from build123d import *

# Parameters (mm, degrees)
SKETCH2_W             = 50
SKETCH2_H             = 50
SKETCH2_R             = 9.525
BOSS_EXTRUDE1_DEPTH   = 6.35
F_4_CLEARANCE_HOLE1_D = 3.2639


with BuildPart() as part:
    # Sketch2 → Boss-Extrude1 (new body)
    with BuildSketch(Plane(origin=(0, 0, 0), x_dir=(1, 0, 0), z_dir=(0, 1, 0))):
        Rectangle(SKETCH2_W, SKETCH2_H)
        Circle(SKETCH2_R, mode=Mode.SUBTRACT)
    extrude(amount=BOSS_EXTRUDE1_DEPTH)

    # #4 Clearance Hole1 (through all)
    with Locations(Plane(origin=(0, 6.35, 0), x_dir=(1, 0, 0), z_dir=(0, 1, 0))):
        with Locations((-21, -21), (21, -21), (21, 21), (-21, 21)):
            Hole(F_4_CLEARANCE_HOLE1_D / 2)


solid = part.part
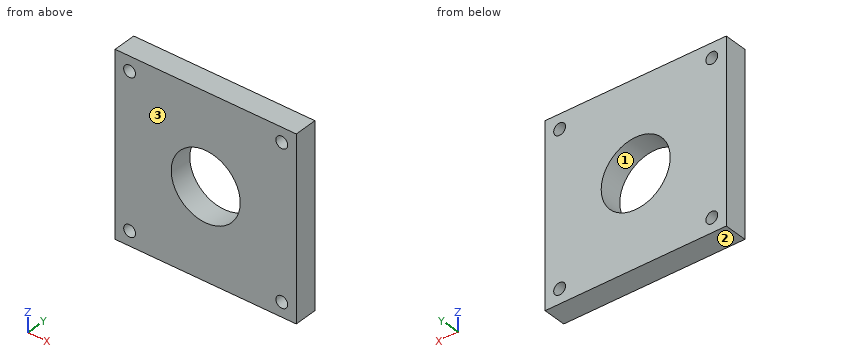
The listing builds one solid part. Answer for the finished solid, in the listing's coordinates (mm). Face numbers are marked on the shaded views. Round coordinates to 2 decimals unless told otherwise and drop trailing zeros. Order: outer loops, then holes, each group sorted by start corner. A loop starts at its lowest first (then second) coordinate and runs counter-clockwise, first axis right, second up. Notation, with made-up numbers: M 9.25,-33 L 65.25,-33 A21 cw 65.25,-6 Z; hole C 55.25,-11 d11. An arc over 180 degrees is marked long. Answer in a Markdown table with one row per item. Add a question column.
1) The part is cut by section C-C on x = 0. Determine the outline of the cut face in (y, z) (3 decimals), plus the area to 3 significant figures.
2) Consider line 1 along X through (y, z) = (2.5, 21); line 2 along Z through (x, y) = (0, 2.75) (3 decimals). Determine where each line is inside the solid, lowest interval first. Write a range as from..to.
3) The part is cut by section D-D on z = 0. Determine the outline of the cut face in (x, y) (3 decimals).
4) The part is cut by section A-A on z = 21. Determine the outline of the cut face in (x, y), plus the area to 3 significant figures.
5) Determine the mould class of the marked faces 1, 2 and 3 for opening direction Z: pulls with the +Z half, pulls with the -Z half, needs draft (parallel to the pull), parting line crosses it, or undercut.
6) The part is cut by section B-B on x = 21. Determine the outline of the cut face in (y, z), plus the area to 3 significant figures.
Findings below:
| question | item | result |
|---|---|---|
| 1 | outline | M 0,-25 L 6.35,-25 L 6.35,-9.525 L 0,-9.525 Z; M 0,9.525 L 6.35,9.525 L 6.35,25 L 0,25 Z |
| 1 | area | 197 mm² |
| 2 | line 1 | x = -25..-22.63, -19.37..19.37, 22.63..25 |
| 2 | line 2 | z = -25..-9.525, 9.525..25 |
| 3 | outline | M -25,0 L -9.525,0 L -9.525,6.35 L -25,6.35 Z; M 9.525,0 L 25,0 L 25,6.35 L 9.525,6.35 Z |
| 4 | outline | M -25,0 L -22.63,0 L -22.63,6.35 L -25,6.35 Z; M -19.37,0 L 19.37,0 L 19.37,6.35 L -19.37,6.35 Z; M 22.63,0 L 25,0 L 25,6.35 L 22.63,6.35 Z |
| 4 | area | 276 mm² |
| 5 | face 1 | undercut |
| 5 | face 2 | pulls with the -Z half |
| 5 | face 3 | needs draft |
| 6 | outline | M 0,-25 L 6.35,-25 L 6.35,-22.63 L 0,-22.63 Z; M 0,-19.37 L 6.35,-19.37 L 6.35,19.37 L 0,19.37 Z; M 0,22.63 L 6.35,22.63 L 6.35,25 L 0,25 Z |
| 6 | area | 276 mm² |
